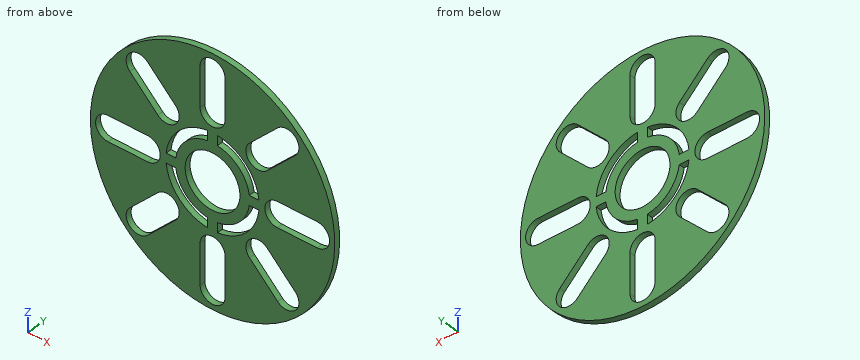
from build123d import *

# Parameters (mm, degrees)
SKETCH1_R           = 63.5
SKETCH1_R_2         = 14.25
BOSS_EXTRUDE1_DEPTH = 3
CUT_EXTRUDE1_DEPTH  = 90.852657167
CIRPATTERN1_COUNT   = 8


with BuildPart() as part:
    # Sketch1 → Boss-Extrude1 (new body)
    with BuildSketch(Plane(origin=(0, 0, 0), x_dir=(1, 0, 0), z_dir=(0, 1, 0))):
        with Locations(Location((0, 0, 0), (0, 0, 270))):
            Circle(SKETCH1_R)
        with Locations(Location((0, 0, 0), (0, 0, 270))):
            Circle(SKETCH1_R_2, mode=Mode.SUBTRACT)
        with BuildLine():
            Line((-2.5, 19.086971997), (-2.5, 24.120789788))
            ThreePointArc((-2.5, 24.120789788), (-17.147339444, 17.147339444), (-24.120789788, 2.5))
            Line((-24.120789788, 2.5), (-19.086971997, 2.5))
            ThreePointArc((-19.086971997, 2.5), (-13.611805538, 13.611805538), (-2.5, 19.086971997))
        make_face(mode=Mode.SUBTRACT)
        with BuildLine():
            Line((2.5, 19.086971997), (2.5, 24.120789788))
            ThreePointArc((2.5, 24.120789788), (17.147339444, 17.147339444), (24.120789788, 2.5))
            Line((24.120789788, 2.5), (19.086971997, 2.5))
            ThreePointArc((19.086971997, 2.5), (13.611805538, 13.611805538), (2.5, 19.086971997))
        make_face(mode=Mode.SUBTRACT)
        with BuildLine():
            Line((19.086971997, -2.5), (24.120789788, -2.5))
            ThreePointArc((24.120789788, -2.5), (17.147339444, -17.147339444), (2.5, -24.120789788))
            Line((2.5, -24.120789788), (2.5, -19.086971997))
            ThreePointArc((2.5, -19.086971997), (13.611805538, -13.611805538), (19.086971997, -2.5))
        make_face(mode=Mode.SUBTRACT)
        with BuildLine():
            Line((-2.5, -19.086971997), (-2.5, -24.120789788))
            ThreePointArc((-2.5, -24.120789788), (-17.147339444, -17.147339444), (-24.120789788, -2.5))
            Line((-24.120789788, -2.5), (-19.086971997, -2.5))
            ThreePointArc((-19.086971997, -2.5), (-13.611805538, -13.611805538), (-2.5, -19.086971997))
        make_face(mode=Mode.SUBTRACT)
    extrude(amount=BOSS_EXTRUDE1_DEPTH)

    # Sketch4 → Cut-Extrude1 (cut, through all)
    with BuildSketch(Plane(origin=(0, 3, 0), x_dir=(1, 0, 0), z_dir=(0, 1, 0))):
        with BuildLine():
            Line((-6.5, 33.7), (-6.5, 54.3))
            ThreePointArc((-6.5, 54.3), (0, 60.8), (6.5, 54.3))
            Line((6.5, 54.3), (6.5, 33.7))
            ThreePointArc((6.5, 33.7), (0, 27.2), (-6.5, 33.7))
        make_face()
    cut_extrude1 = extrude(amount=-CUT_EXTRUDE1_DEPTH, mode=Mode.SUBTRACT)

    # CirPattern1: Cut-Extrude1 ×8 about axis
    cirpattern1_axis = Axis((0, 0, 0), (0, 1, 0))
    for i in range(1, CIRPATTERN1_COUNT):
        add(cut_extrude1.rotate(cirpattern1_axis, i * 360 / CIRPATTERN1_COUNT), mode=Mode.SUBTRACT)


solid = part.part
Geometry: final body of the model. Coordinates: model frame, mm. Coordinates: 2 decimals unless noted, no trailing zeros. Order: outer loops, then holes, each group sorted by start corner. A loop starts at its lowest first (then second) coordinate and runs counter-clockwise, first axis right, second up.
1) Section C-C (z = -51). Return loops of the section in (x, y), then the cut area to 3 significant figures.
Result sheet:
outline: (-37.83, 0) - (-6.5, 0) - (-6.5, 3) - (-37.83, 3) - close; (6.5, 0) - (37.83, 0) - (37.83, 3) - (6.5, 3) - close
area: 188 mm2
2) Ray query, probe 1 along X at (y, z) = (1.7, 0); probe 2 along Z at (x, y) = (12, 2.3); probe 3 along X at (y, z) = (1.5, -41). Return the intervals inside material, ascending.
Result sheet:
probe 1: x = -63.5 to -60.8, -27.2 to -14.25, 14.25 to 27.2, 60.8 to 63.5
probe 2: z = -62.36 to -21.07, -15.05 to -7.69, 7.69 to 15.05, 21.07 to 62.36
probe 3: x = -48.49 to -44.35, -31.81 to -6.5, 6.5 to 31.81, 44.35 to 48.49
3) First-contact query: P1, Ø1.5, axis at y = 2, z = 22.5, coming from the +X side; P2, Ø1.5, axis at x = 4, y = 1.5, coming from the -Z side; P3, Ø1.5, axis at x = 9, y = 1.5, coming from the -Z side. Flat tips, straight axial feed; report the tip coordinate or a pass-through.
Result sheet:
P1: stops at x = 59.66
P2: stops at z = -63.42
P3: stops at z = -62.96
4) Section B-B (x = 40.5). Return loops of the section in (y, z), then the cut area to 3 significant figures.
Result sheet:
outline: (0, -48.91) - (3, -48.91) - (3, -44.55) - (0, -44.55) - close; (0, -31.31) - (3, -31.31) - (3, -6.5) - (0, -6.5) - close; (0, 6.5) - (3, 6.5) - (3, 31.31) - (0, 31.31) - close; (0, 44.55) - (3, 44.55) - (3, 48.91) - (0, 48.91) - close
area: 175 mm2
5) Section D-D (y = 0.7). Give the number of separate pieces and of enclosed holes in the cut face, then the cut area to 3 significant figures.
Result sheet:
separate pieces: 1
enclosed holes: 13
area: 8,240 mm2
6) Section A-A (z = 0). Return loops of the section in (x, y), then the cut area to 3 significant figures.
Result sheet:
outline: (-63.5, 0) - (-60.8, 0) - (-60.8, 3) - (-63.5, 3) - close; (-27.2, 0) - (-14.25, 0) - (-14.25, 3) - (-27.2, 3) - close; (14.25, 0) - (27.2, 0) - (27.2, 3) - (14.25, 3) - close; (60.8, 0) - (63.5, 0) - (63.5, 3) - (60.8, 3) - close
area: 93.9 mm2
